Build history of the part. All positions in model axes, mm. A direction names the side the tool comes from. Coordinates: 2 decimals unless noted, no trailing zeros. Write each loop counter-clockwise with the first axis right and the second up, starting at its lowest first coordinate (ties: lowest second). Pieces come first, ordered by that corner, then holes.
```python
from build123d import *

# Parameters (mm, degrees)
SKETCH1_W           = 10
SKETCH1_H           = 10
SKETCH1_R           = 3.5
BOSS_EXTRUDE1_DEPTH = 2
SKETCH1_2_R         = 3.5
BOSS_EXTRUDE2_DEPTH = 10
BOSS_EXTRUDE4_START = 8
SKETCH1_4_W         = 10
SKETCH1_4_H         = 10
SKETCH1_4_R         = 3.5
BOSS_EXTRUDE4_DEPTH = 2
SKETCH2_R           = 2.330446687
CUT_EXTRUDE1_DEPTH  = 18.320508076


with BuildPart() as part:
    # Sketch1 → Boss-Extrude1 (new body)
    with BuildSketch(Plane(origin=(0, 0, 0), x_dir=(1, 0, 0), z_dir=(0, 1, 0))):
        with Locations((5, -5)):
            Rectangle(SKETCH1_W, SKETCH1_H)
        with Locations(Location((5, -5, 0), (0, 0, 270))):
            Circle(SKETCH1_R, mode=Mode.SUBTRACT)
    extrude(amount=BOSS_EXTRUDE1_DEPTH)

    # Sketch1<2> → Boss-Extrude2 (add)
    with BuildSketch(Plane(origin=(0, 0, 0), x_dir=(1, 0, 0), z_dir=(0, 1, 0))):
        with Locations(Location((5, -5, 0), (0, 0, 270))):
            Circle(SKETCH1_2_R)
    extrude(amount=BOSS_EXTRUDE2_DEPTH)

    # Sketch1<4> → Boss-Extrude4 (add)
    with BuildSketch(Plane(origin=(0, 0, 0), x_dir=(1, 0, 0), z_dir=(0, 1, 0)).offset(BOSS_EXTRUDE4_START)):
        with Locations((5, -5)):
            Rectangle(SKETCH1_4_W, SKETCH1_4_H)
        with Locations(Location((5, -5, 0), (0, 0, 270))):
            Circle(SKETCH1_4_R, mode=Mode.SUBTRACT)
    extrude(amount=BOSS_EXTRUDE4_DEPTH)

    # Sketch2 → Cut-Extrude1 (cut, through all)
    with BuildSketch(Plane(origin=(0, 10, 0), x_dir=(1, 0, 0), z_dir=(0, 1, 0))):
        with Locations(Location((5, -5, 0), (0, 0, 270))):
            Circle(SKETCH2_R)
    extrude(amount=-CUT_EXTRUDE1_DEPTH, mode=Mode.SUBTRACT)


solid = part.part
```
1. Saw through at C-C on y = 0.75. List the corners of the cut face in (x, z), plus the area to 3 significant figures.
Computed values:
outline: (0, 0) - (10, 0) - (10, 10) - (0, 10) - close; hole circle Ø4.66 at (5, 5)
area: 82.9 mm2
2. Saw through at D-D on z = 9.25. List the corners of the cut face in (x, y).
Computed values:
outline: (0, 0) - (10, 0) - (10, 2) - (0, 2) - close; (0, 8) - (10, 8) - (10, 10) - (0, 10) - close
3. Saw through at A-A on x = 5. List the corners of the cut face in (y, z), plus the area to 3 significant figures.
Computed values:
outline: (0, 0) - (2, 0) - (2, 1.5) - (8, 1.5) - (8, 0) - (10, 0) - (10, 2.67) - (0, 2.67) - close; (0, 7.33) - (10, 7.33) - (10, 10) - (8, 10) - (8, 8.5) - (2, 8.5) - (2, 10) - (0, 10) - close
area: 35.4 mm2
4. Flat gauge pins, fed straight in: pin 1 (2 mm diameter, centred on y = 6.5, z = 2.5, fed in from -X); pin 2 (3 mm diameter, centred on x = 3.5, y = 5, fed in from +Z); pin 3 (3.5 mm diameter, centred on x = 5, z = 5, fed in from -Y). Where does each tip first touch, or does it go through?
Computed values:
pin 1: stops at x = 1.84
pin 2: stops at z = 8.5
pin 3: passes through
5. Mould opens along Y. For faces 1 (the face through (7.2, 10, 3.8)), 2 (the face through (5, 9, 0)), 3 (the face through (2.7, 8, 1.6)) say: +Y half, -Y half, draft (parallel to the pull), parting line (faces both ways), or undercut.
Computed values:
face 1: +Y half
face 2: draft
face 3: undercut
6. Probe line 1 along Y through (x, z) = (1, 2); line 2 along X through (y, z) = (2.75, 5); line 3 along X through (y, z) = (3.75, 4.25). List the from-to ranges inside material, lowest first.
Computed values:
line 1: y = 0 to 2, 8 to 10
line 2: x = 1.5 to 2.67, 7.33 to 8.5
line 3: x = 1.58 to 2.79, 7.21 to 8.42
7. Saw through at B-B on z = 5. List the corners of the cut face in (x, y).
Computed values:
outline: (0, 0) - (2.67, 0) - (2.67, 10) - (0, 10) - (0, 8) - (1.5, 8) - (1.5, 2) - (0, 2) - close; (7.33, 0) - (10, 0) - (10, 2) - (8.5, 2) - (8.5, 8) - (10, 8) - (10, 10) - (7.33, 10) - close
8. 3-axis set-ups, long thin cutter, end or side, ignore diameter. For faces 4 (the face through (0, 1, 5)), 5 (the face through (3.659, 4.958, 8.233)): which of +Z, -Z, +X, -X, +Y, -Y reach the whole face in a straight line?
Computed values:
face 4: +Z, -Z, -X, +Y, -Y
face 5: none
